```python
from build123d import *

# Parameters (mm, degrees)
SKETCH_1_W      = 180
SKETCH_1_H      = 50
SKETCH_1_R      = 1.5
SKETCH_1_R_2    = 1.25
EXTRUDE_1_DEPTH = 2


with BuildPart() as part:
    # 草图1 → 凸台-拉伸1 (new body)
    with BuildSketch(Plane(origin=(0, 0, 0), x_dir=(1, 0, 0), z_dir=(0, 1, 0))):
        with Locations((90, -25)):
            Rectangle(SKETCH_1_W, SKETCH_1_H)
        with Locations(Location((9, -11.5, 0), (0, 0, 270))):
            Circle(SKETCH_1_R, mode=Mode.SUBTRACT)
        with Locations(Location((9, -38.5, 0), (0, 0, 270))):
            Circle(SKETCH_1_R, mode=Mode.SUBTRACT)
        with Locations(Location((24, -11.5, 0), (0, 0, 270))):
            Circle(SKETCH_1_R, mode=Mode.SUBTRACT)
        with Locations(Location((24, -38.5, 0), (0, 0, 270))):
            Circle(SKETCH_1_R, mode=Mode.SUBTRACT)
        with Locations(Location((30, -38.5, 0), (0, 0, 270))):
            Circle(SKETCH_1_R, mode=Mode.SUBTRACT)
        with Locations(Location((45, -38.5, 0), (0, 0, 270))):
            Circle(SKETCH_1_R, mode=Mode.SUBTRACT)
        with Locations(Location((45, -11.5, 0), (0, 0, 270))):
            Circle(SKETCH_1_R, mode=Mode.SUBTRACT)
        with Locations(Location((30, -11.5, 0), (0, 0, 270))):
            Circle(SKETCH_1_R, mode=Mode.SUBTRACT)
        with Locations(Location((51, -38.5, 0), (0, 0, 270))):
            Circle(SKETCH_1_R, mode=Mode.SUBTRACT)
        with Locations(Location((66, -38.5, 0), (0, 0, 270))):
            Circle(SKETCH_1_R, mode=Mode.SUBTRACT)
        with Locations(Location((66, -11.5, 0), (0, 0, 270))):
            Circle(SKETCH_1_R, mode=Mode.SUBTRACT)
        with Locations(Location((51, -11.5, 0), (0, 0, 270))):
            Circle(SKETCH_1_R, mode=Mode.SUBTRACT)
        with Locations(Location((72, -38.5, 0), (0, 0, 270))):
            Circle(SKETCH_1_R, mode=Mode.SUBTRACT)
        with Locations(Location((87, -38.5, 0), (0, 0, 270))):
            Circle(SKETCH_1_R, mode=Mode.SUBTRACT)
        with Locations(Location((87, -11.5, 0), (0, 0, 270))):
            Circle(SKETCH_1_R, mode=Mode.SUBTRACT)
        with Locations(Location((72, -11.5, 0), (0, 0, 270))):
            Circle(SKETCH_1_R, mode=Mode.SUBTRACT)
        with Locations(Location((93, -38.5, 0), (0, 0, 270))):
            Circle(SKETCH_1_R, mode=Mode.SUBTRACT)
        with Locations(Location((108, -38.5, 0), (0, 0, 270))):
            Circle(SKETCH_1_R, mode=Mode.SUBTRACT)
        with Locations(Location((108, -11.5, 0), (0, 0, 270))):
            Circle(SKETCH_1_R, mode=Mode.SUBTRACT)
        with Locations(Location((93, -11.5, 0), (0, 0, 270))):
            Circle(SKETCH_1_R, mode=Mode.SUBTRACT)
        with Locations(Location((114, -38.5, 0), (0, 0, 270))):
            Circle(SKETCH_1_R, mode=Mode.SUBTRACT)
        with Locations(Location((129, -38.5, 0), (0, 0, 270))):
            Circle(SKETCH_1_R, mode=Mode.SUBTRACT)
        with Locations(Location((129, -11.5, 0), (0, 0, 270))):
            Circle(SKETCH_1_R, mode=Mode.SUBTRACT)
        with Locations(Location((114, -11.5, 0), (0, 0, 270))):
            Circle(SKETCH_1_R, mode=Mode.SUBTRACT)
        with Locations(Location((135, -38.5, 0), (0, 0, 270))):
            Circle(SKETCH_1_R, mode=Mode.SUBTRACT)
        with Locations(Location((150, -38.5, 0), (0, 0, 270))):
            Circle(SKETCH_1_R, mode=Mode.SUBTRACT)
        with Locations(Location((150, -11.5, 0), (0, 0, 270))):
            Circle(SKETCH_1_R, mode=Mode.SUBTRACT)
        with Locations(Location((135, -11.5, 0), (0, 0, 270))):
            Circle(SKETCH_1_R, mode=Mode.SUBTRACT)
        with Locations(Location((156, -38.5, 0), (0, 0, 270))):
            Circle(SKETCH_1_R, mode=Mode.SUBTRACT)
        with Locations(Location((171, -38.5, 0), (0, 0, 270))):
            Circle(SKETCH_1_R, mode=Mode.SUBTRACT)
        with Locations(Location((171, -11.5, 0), (0, 0, 270))):
            Circle(SKETCH_1_R, mode=Mode.SUBTRACT)
        with Locations(Location((156, -11.5, 0), (0, 0, 270))):
            Circle(SKETCH_1_R, mode=Mode.SUBTRACT)
        with Locations(Location((2, -2, 0), (0, 0, 270))):
            Circle(SKETCH_1_R_2, mode=Mode.SUBTRACT)
        with Locations(Location((78, -2, 0), (0, 0, 270))):
            Circle(SKETCH_1_R_2, mode=Mode.SUBTRACT)
        with Locations(Location((2, -28, 0), (0, 0, 270))):
            Circle(SKETCH_1_R_2, mode=Mode.SUBTRACT)
        with Locations(Location((78, -28, 0), (0, 0, 270))):
            Circle(SKETCH_1_R_2, mode=Mode.SUBTRACT)
    extrude(amount=EXTRUDE_1_DEPTH)


solid = part.part
```
Build history of the part. All positions in model axes, mm. Give positions to 0.01 mm unless a question says otherwise; leave off trailing zeros. Loops run counter-clockwise (first coordinate to the right, second up) from the corner with the lowest first, then second, coordinate; pieces in that order, holes last. Notation, with made-up numbers: (37, -14.5) -> (77, -14.5) arc R16 ccw to (77, 5.5) -> close; hole circle Ø3 at (25.25, 88.25). An arc over 180 degrees is marked (long way). One line per question, with ' | ' between items.
Q1. Cut at A-A, the plane x = 108. Write the cut outline in (y, z).
Filled sheet:
outline: (0, 0) -> (2, 0) -> (2, 10) -> (0, 10) -> close; (0, 13) -> (2, 13) -> (2, 37) -> (0, 37) -> close; (0, 40) -> (2, 40) -> (2, 50) -> (0, 50) -> close
Q2. Cut at B-B, the plane y = 1.5. Count the separate pieces of the cut face and the enclosed holes in it, plus the area to 3 significant figures.
Filled sheet:
separate pieces: 1 | enclosed holes: 36 | area: 8,750 mm²
Q3. Pull direction X, two halves, no side cores. Call faces 1 (the flat face through (89, 0, 25)), 2 (the cylindrical face through (115.487, 0.986, 38.305)): pulls with the +X half, pulls with the -X half, needs draft (parallel to the pull), parting line crosses it, or undercut.
Filled sheet:
face 1: needs draft | face 2: undercut
Q4. Drop a flat-ended pin along its axis: pin 1 (2.5 mm diameter, centred on x = 150, z = 38.5, fed in from +Y). Give the stop position or say it passes through.
Filled sheet:
pin 1: passes through
Q5. Drill centre lines: line 1 along Z through (x, y) = (156, 0.65); line 2 along X through (y, z) = (0.6, 28); line 3 along Z through (x, y) = (23.5, 0.15). Where is each one in solid material? Low to high. Write a range as [from, to].
Filled sheet:
line 1: z = [0, 10], [13, 37], [40, 50] | line 2: x = [0, 0.75], [3.25, 76.75], [79.25, 180] | line 3: z = [0, 10.09], [12.91, 37.09], [39.91, 50]
